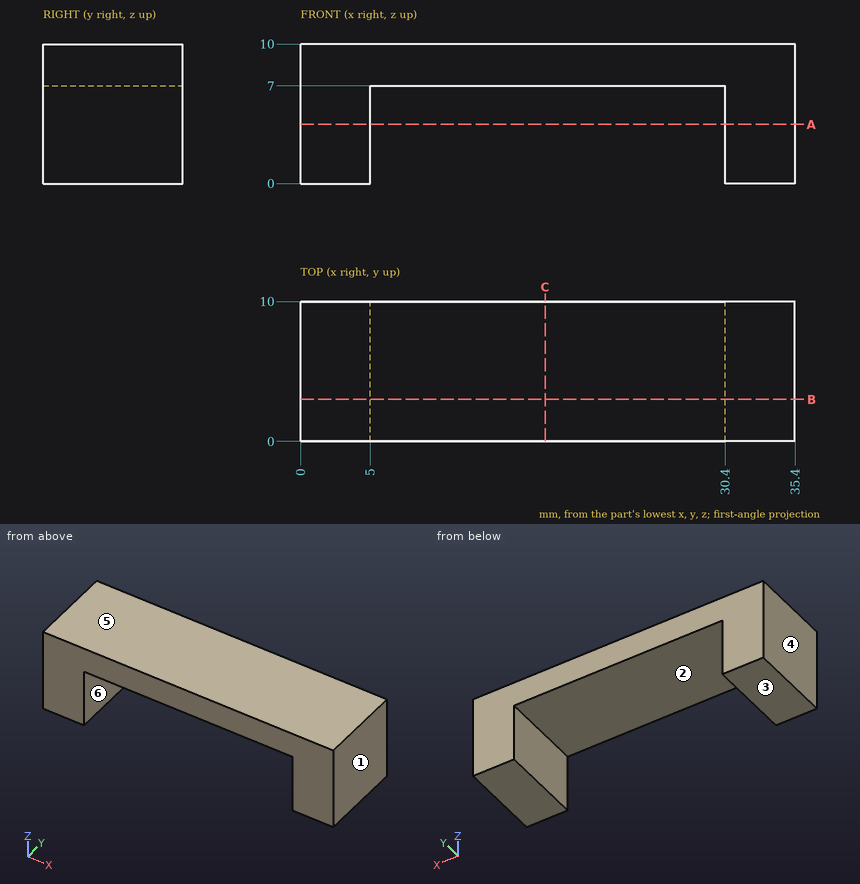
Job drawing, mm, ordinate dimensions from the low corner. One solid piece. A direction names the side the tool comes from. Give positions to 0.01 mm unless a question says otherwise; leave off trailing zeros. Loops run counter-clockwise (first coordinate to the right, second up) from the corner with the lowest first, then second, coordinate; pieces in that order, holes last. Notation, with made-up numbers: (86.25, -23.75) -> (99.25, -23.75) arc R8 cw to (99.25, -19.75) -> close; hole circle Ø9 at (26, -27.75). An arc over 180 degrees is marked (long way). Write each question's results on one line, items separated by ' | '. Start each with the question number.
Q1. Which spindle directions (+Z, -Z, +X, -X, +Y, -Y) get a long thin tool onto all of the face, cutting with end or side? Do the marked faces 5 and 6. Say none if no direction does.
Q2. Wall check: L1, parallel to X at y = 8.5, z = 1.5; L2, parallel to Z at x = 27.5, y = 5.25. Give the ranges that are in metal, low to high.
Q3. Band-saw the part on B-B on y = 3. List the corners of the cut face in (x, z).
Q4. Band-saw the part on C-C on x = 17.5. List the corners of the cut face in (y, z), plus the area to 3 significant figures.
Q5. Pin check, flat tips, straight feed: P1, Ø1.5, axis at x = 19.5, z = 5, coming from the +Y side; P2, Ø5, axis at x = 14, y = 6, coming from the -Z side. Stop position of each tip, or through.
Q6. Band-saw the part on A-A on z = 4.25. List the corners of the cut face in (x, y), plus the area to 3 significant figures.
Q7. Pull direction X, two halves, no side cores. Call the marked faces 1, 2, 3 and 4: +X half, -X half, draft (parallel to the pull), parting line (faces both ways), or undercut.
Results are:
1) face 5: +Z, +X, -X, +Y, -Y | face 6: -Z, +Y, -Y
2) L1: x = 0 to 5, 30.4 to 35.4 | L2: z = 7 to 10
3) outline: (0, 0) -> (5, 0) -> (5, 7) -> (30.4, 7) -> (30.4, 0) -> (35.4, 0) -> (35.4, 10) -> (0, 10) -> close
4) outline: (0, 7) -> (10, 7) -> (10, 10) -> (0, 10) -> close | area: 30.0 mm²
5) P1: passes through | P2: stops at z = 7
6) outline: (0, 0) -> (5, 0) -> (5, 10) -> (0, 10) -> close; (30.4, 0) -> (35.4, 0) -> (35.4, 10) -> (30.4, 10) -> close | area: 100 mm²
7) face 1: +X half | face 2: undercut | face 3: draft | face 4: -X half
